CAD build for the part. Positions are in the model's coordinates, mm. A direction names the side the tool comes from. Coordinates: 2 decimals unless noted, no trailing zeros. Loops run counter-clockwise (first coordinate to the right, second up) from the corner with the lowest first, then second, coordinate; pieces in that order, holes last. Notation, with made-up numbers: (51.5, 12) -> (86.5, 12) arc R35 cw to (86.5, 48) -> close; hole circle Ø1 at (57.25, -30). An arc over 180 degrees is marked (long way). Return JSON: item names as keys, results as strings. Group by question number.
(1) Saw through at D-D on x = -13.5. Write the cut outline in (y, z) (3 decimals).
(2) Saw through at C-C on z = 8. Write the cut outline in (x, y) (1 decimal).
(3) Saw through at B-B on x = 0. Write the cut outline in (y, z) (1 decimal), then the cut area to 3 significant figures.
(4) Probe L1, parallel to Z at x = -15.85, y = 0 (3 decimals); L2, parallel to Y at x = 0, z = 30 (3 decimals); L3, parallel to X at y = 0, z = 28.75 (1 decimal). List the from-to ranges inside material, lowest first.
(5) Flat gauge pins, fed straight in: pin 1 Ø8.5 at (x, y) = (0, 0) entering from +Z; pin 2 Ø2.5 at (y, z) = (0, 40) entering from -X; pin 3 Ø6.5 at (x, y) = (-1, 4.5) entering from -Z. Where does each tip first touch, or does it go through?
(6) Mould opens along X. For faces 4 (the face through (0, 12.7, 23)), 5 (the face through (-17.173, 12.394, 24.146)), 6 (the face through (4.543, 1.431, 40.675)) say: pulls with the +X half, pulls with the -X half, needs draft (parallel to the pull), parting line crosses it, or undercut.
(7) Tool access for faces 1 (the face through (0, -12.7, 23)), 2 (the face through (-4.4, -2.3, 33.528)), 3 (the face through (-15.209, -1.182, 38.329)): list every direction of +Z, -Z, +X, -X, +Y, -Y with a clear straight run to the whole face (end or side of a thin tool).
(8) Saw through at A-A on y = 0. Give the number of separate pieces and of enclosed holes in the cut face, then the cut area to 3 significant figures.
```python
from build123d import *

# Parameters (mm, degrees)
F0_W      = 34.925
F0_H      = 25.4
F1_DEPTH  = 47.625
F2_R      = 11.1125
F3_DEPTH  = 25.4
F4_R      = 9.525
F5_DEPTH  = 8.128
F6_R      = 4.7625
F7_DEPTH  = 25.4
F8_R      = 1.9304
F9_DEPTH  = 16.77604
F10_R     = 1.016
F11_R     = 2.560992
F12_DEPTH = 4.572


with BuildPart() as f1:
    # F0 (on Top) → F1 (new body)
    with BuildSketch(Plane.XY):
        Rectangle(F0_W, F0_H)
    extrude(amount=F1_DEPTH)

    # F2 (on Top) → F3 (cut)
    with BuildSketch(Plane.XY):
        Circle(F2_R)
    extrude(amount=F3_DEPTH, mode=Mode.SUBTRACT)

    # F4 (on face) → F5 (cut)
    with BuildSketch(Plane(origin=(0, 0, 25.4), x_dir=(1, 0, 0), z_dir=(0, 0, -1))):
        Circle(F4_R)
    extrude(amount=-F5_DEPTH, mode=Mode.SUBTRACT)

    # F6 (on face) → F7 (cut)
    with BuildSketch(Plane.XY.offset(47.625)):
        Circle(F6_R)
    extrude(amount=-F7_DEPTH, mode=Mode.SUBTRACT)

    # F8 (on face) → F9 (cut)
    with BuildSketch(Plane(origin=(-17.4625, 0, 0), x_dir=(0, -1, 0), z_dir=(-1, 0, 0))):
        with Locations((0, 21.336)):
            Circle(F8_R)
        with Locations((0, 5.08)):
            Circle(F8_R)
        with Locations((0, 40.600542)):
            Circle(F8_R)
    extrude(amount=-F9_DEPTH, mode=Mode.SUBTRACT)

    # F10
    f10_edges = [f1.edges().sort_by_distance(p)[0] for p in [
        (-17.4625, -12.7, 23.8125),
        (17.4625, -12.7, 23.8125),
        (-17.4625, 12.7, 23.8125),
        (17.4625, 12.7, 23.8125),
    ]]
    fillet(f10_edges, radius=F10_R)

    # F11 (on face) → F12 (cut)
    with BuildSketch(Plane(origin=(-17.4625, 0, 0), x_dir=(0, -1, 0), z_dir=(-1, 0, 0))):
        with Locations((0, 40.600542)):
            Circle(F11_R)
    extrude(amount=-F12_DEPTH, mode=Mode.SUBTRACT)


solid = f1.part
```
Geometry results:
{
 "1": {"outline": "(-12.7, 0) -> (12.7, 0) -> (12.7, 47.625) -> (-12.7, 47.625) -> close; hole circle Ø5.122 at (0, 40.601); hole circle Ø3.861 at (0, 5.08); hole circle Ø3.861 at (0, 21.336)"},
 "2": {"outline": "(-17.5, -11.7) arc R1 ccw to (-16.4, -12.7) -> (16.4, -12.7) arc R1 ccw to (17.5, -11.7) -> (17.5, 11.7) arc R1 ccw to (16.4, 12.7) -> (-16.4, 12.7) arc R1 ccw to (-17.5, 11.7) -> close; hole circle Ø22.2 at (0, 0)"},
 "3": {"outline": "(-12.7, 0) -> (-11.1, 0) -> (-11.1, 25.4) -> (-9.5, 25.4) -> (-9.5, 33.5) -> (-4.8, 33.5) -> (-4.8, 47.6) -> (-12.7, 47.6) -> close; (4.8, 33.5) -> (9.5, 33.5) -> (9.5, 25.4) -> (11.1, 25.4) -> (11.1, 0) -> (12.7, 0) -> (12.7, 47.6) -> (4.8, 47.6) -> close", "area": "356 mm²"},
 "4": {"L1": "0 to 3.15, 7.01 to 19.406, 23.266 to 38.04, 43.162 to 47.625", "L2": "-12.7 to -9.525, 9.525 to 12.7", "L3": "-17.5 to -9.5, 9.5 to 17.5"},
 "5": {"pin 1": "through", "pin 2": "x = 4.6", "pin 3": "z = 33.53"},
 "6": {"face 4": "needs draft", "face 5": "pulls with the -X half", "face 6": "undercut"},
 "7": {"face 1": "+Z, -Z, +X, -X, -Y", "face 2": "-Z", "face 3": "-X"},
 "8": {"separate pieces": "5", "enclosed holes": "0", "area": "706 mm²"}
}
